Read the model definition and answer for the solid it produces. Units are mm, in the model's axes. A direction names the side the tool comes from. Coordinates: 2 decimals unless noted, no trailing zeros. Loops run counter-clockwise (first coordinate to the right, second up) from the corner with the lowest first, then second, coordinate; pieces in that order, holes last. Notation, with made-up numbers: M -3,-15 L 49,-15 A30 cw 49,17 Z; hole C 53,36.5 d7. An arc over 180 degrees is marked long. One line per item, written item: value. Start each with the question number.
1. The part is cut by section B-B (x = 6.5). Write down the section's boundary in (y, z), then the cut area to 3 significant figures.
2. Consider probe 1 along Z at (x, y) = (-15, -6.5); probe 2 along Y at (x, z) = (0, 8); probe 3 along X at (y, z) = (-16.5, 3). Determine where each line is inside the solid, lowest interval first.
3. Flat-ended cylindrical pins translate along their axes: pin 1 (22 mm diameter, centred on x = 23.5, z = 33.5, fed in from +Y); pin 2 (4 mm diameter, centred on y = -2, z = 17, fed in from -X); pin 3 (9 mm diameter, centred on x = 24, y = -0.5, fed in from +Z). Find the tip coordinate at first contact, or state that the pin passes through.
4. The part is cut by section D-D (z = 24.5). Write down the section's boundary in (x, y), then the cut area to 3 significant figures.
5. Determine the mould class of faces 1 (the face through (-2.17, -9.76, 9.86)), 2 (the face through (10, -4, 0)), 3 (the face through (40, -15, 20)) for opening direction X: +X half, -X half, draft (parallel to the pull), parting line (faces both ways), or undercut.
6. The part is cut by section C-C (x = 13.5). Write down the section's boundary in (y, z).
7. The part is cut by section A-A (z = 15). Write down the section's boundary in (x, y), then the cut area to 3 significant figures.
8. For faces 4 (the face through (25, 0, 10)), 5 (the face through (-20, -9, 10)), 6 (the face through (10, -15, 40)), 7 (the face through (10, -10, 30)), determine the directions among +Z, -Z, +X, -X, +Y, -Y from which every point of the face is accessible in a straight line to the end or side of a thin tool.
```python
from build123d import *

# Parameters (mm, degrees)
SKETCH1_R           = 10
BOSS_EXTRUDE1_DEPTH = 20
BOSS_EXTRUDE2_DEPTH = 20


with BuildPart() as part:
    # Sketch1 → Boss-Extrude1 (new body)
    with BuildSketch(Plane.XY):
        with BuildLine():
            Line((-20, 0), (-20, -10))
            Line((-20, -10), (-20, -19.161425494))
            Line((-20, -19.161425494), (40, -20))
            Line((40, -20), (40, -10))
            ThreePointArc((40, -10), (37.071067812, -2.928932188), (30, 0))
            Line((30, 0), (20, 0))
            ThreePointArc((20, 0), (0, 20), (-20, 0))
        make_face()
        Circle(SKETCH1_R, mode=Mode.SUBTRACT)
    extrude(amount=BOSS_EXTRUDE1_DEPTH)

    # Sketch3 → Boss-Extrude2 (add)
    with BuildSketch(Plane.XY.offset(20)):
        Polygon((-20.104236771, -10), (40, -10), (40, -20), (-20, -19.161425494), align=None)
    extrude(amount=BOSS_EXTRUDE2_DEPTH)


solid = part.part
```
Answer block:
1. outline: M -19.53,0 L -7.6,0 L -7.6,20 L -10,20 L -10,40 L -19.53,40 Z; M 7.6,0 L 18.91,0 L 18.91,20 L 7.6,20 Z
1. area: 656 mm2
2. probe 1: z = 0 to 20
2. probe 2: y = -19.44 to -10, 10 to 20
2. probe 3: x = -20 to 40
3. pin 1: stops at y = -10
3. pin 2: stops at x = -20
3. pin 3: stops at z = 20
4. outline: M -20.1,-10 L -20,-19.16 L 40,-20 L 40,-10 Z
4. area: 575 mm2
5. face 1: undercut
5. face 2: draft
5. face 3: +X half
6. outline: M -19.63,0 L 14.76,0 L 14.76,20 L -10,20 L -10,40 L -19.63,40 Z
7. outline: M -20,-19.16 L 40,-20 L 40,-10 A10 ccw 30,0 L 20,0 A20 ccw -20,0 Z; hole C 0,0 d20
7. area: 1,470 mm2
8. face 4: +Z, -Z, +X, +Y
8. face 5: -Z, -X, +Y, -Y
8. face 6: +Z, +X, -X, +Y, -Y
8. face 7: +Z, +X, -X, +Y
